Geometry check sheet. Reference: the model listing, model coordinates, mm. A direction names the side the tool comes from. Give positions to 0.01 mm unless a question says otherwise; leave off trailing zeros. Order: outer loops, then holes, each group sorted by start corner. A loop starts at its lowest first (then second) coordinate and runs counter-clockwise, first axis right, second up. Notation, with made-up numbers: M -30.75,76 L -11.75,76 A16 cw -11.75,91 Z; hole C -6.75,7 d11. An arc over 180 degrees is marked long. Answer as CSV lines item,"result".
from build123d import *

# Parameters (mm, degrees)
BOSS_EXTRUDE1_DEPTH = 21
BOSS_EXTRUDE2_DEPTH = 14
SKETCH6_R           = 2
CUT_EXTRUDE6_DEPTH  = 5
SKETCH7_R           = 2
CUT_EXTRUDE7_DEPTH  = 5


with BuildPart() as part:
    # Sketch2 → Boss-Extrude1 (new body)
    with BuildSketch(Plane.XY):
        with BuildLine():
            Line((-24, 0), (-14, 0))
            ThreePointArc((-14, 0), (-12.585786438, 0.585786438), (-12, 2))
            Line((-12, 2), (-12, 14))
            ThreePointArc((-12, 14), (-11.414213562, 15.414213562), (-10, 16))
            Line((-10, 16), (0, 16))
            Line((0, 16), (10, 16))
            ThreePointArc((10, 16), (11.414213562, 15.414213562), (12, 14))
            Line((12, 14), (12, 2))
            ThreePointArc((12, 2), (12.585786438, 0.585786438), (14, 0))
            Line((14, 0), (24, 0))
            Line((24, 0), (24, 2))
            Line((24, 2), (15, 2))
            ThreePointArc((15, 2), (14.292893219, 2.292893219), (14, 3))
            Line((14, 3), (14, 14))
            ThreePointArc((14, 14), (12.828427125, 16.828427125), (10, 18))
            Line((10, 18), (0, 18))
            Line((0, 18), (-10, 18))
            ThreePointArc((-10, 18), (-12.828427125, 16.828427125), (-14, 14))
            Line((-14, 14), (-14, 3))
            ThreePointArc((-14, 3), (-14.292893219, 2.292893219), (-15, 2))
            Line((-15, 2), (-24, 2))
            Line((-24, 2), (-24, 0))
        make_face()
    extrude(amount=BOSS_EXTRUDE1_DEPTH)

    # Sketch3 → Boss-Extrude2 (add)
    with BuildSketch(Plane.XY.offset(21)):
        with BuildLine():
            Line((-14, 3), (-12, 2))
            ThreePointArc((-12, 2), (-12.585786438, 0.585786438), (-14, 0))
            Line((-14, 0), (-24, 0))
            Line((-24, 0), (-24, 2))
            Line((-24, 2), (-15, 2))
            ThreePointArc((-15, 2), (-14.292893219, 2.292893219), (-14, 3))
        make_face()
        with BuildLine():
            Line((12, 2), (14, 3))
            ThreePointArc((14, 3), (14.292893219, 2.292893219), (15, 2))
            Line((15, 2), (24, 2))
            Line((24, 2), (24, 0))
            Line((24, 0), (14, 0))
            ThreePointArc((14, 0), (12.585786438, 0.585786438), (12, 2))
        make_face()
    extrude(amount=BOSS_EXTRUDE2_DEPTH)

    # Sketch6 → Cut-Extrude6 (cut)
    with BuildSketch(Plane(origin=(0, 0, 0), x_dir=(1, 0, 0), z_dir=(0, 1, 0))):
        with Locations(Location((-19, -5, 0), (0, 0, 90))):
            Circle(SKETCH6_R)
        with Locations(Location((-19, -30, 0), (0, 0, 90))):
            Circle(SKETCH6_R)
        with Locations(Location((19, -30, 0), (0, 0, 90))):
            Circle(SKETCH6_R)
        with Locations(Location((19, -5, 0), (0, 0, 90))):
            Circle(SKETCH6_R)
    extrude(amount=CUT_EXTRUDE6_DEPTH, mode=Mode.SUBTRACT)

    # Sketch7 → Cut-Extrude7 (cut)
    with BuildSketch(Plane(origin=(0, 18, 0), x_dir=(1, 0, 0), z_dir=(0, 1, 0))):
        with Locations(Location((0, -8, 0), (0, 0, 270))):
            Circle(SKETCH7_R)
        with Locations(Location((0, -16, 0), (0, 0, 270))):
            Circle(SKETCH7_R)
    extrude(amount=-CUT_EXTRUDE7_DEPTH, mode=Mode.SUBTRACT)


solid = part.part
(1) Section check B-B on x = 0. Enter the section's corners in (y, z), then the cut area to 3 significant figures.
The answers:
outline,"M 16,0 L 18,0 L 18,6 L 16,6 Z; M 16,10 L 18,10 L 18,14 L 16,14 Z; M 16,18 L 18,18 L 18,21 L 16,21 Z"
area,"26.0 mm2"
(2) Gauge pin test, flat ends, axial feed: P1, Ø7, axis at x = 21.5, z = 15, coming from the +Y side; P2, Ø3.5, axis at y = 9, z = 11, coming from the +X side; P3, Ø6, axis at x = -1.5, z = 8, coming from the -Y side; P4, Ø2.5, axis at x = 19, z = 5, coming from the +Y side. Record the tip position at first contact, or that the pin passes through.
The answers:
P1,"stops at y = 2"
P2,"stops at x = 14"
P3,"stops at y = 16"
P4,"passes through"
(3) Section check D-D on y = 6.75. Enter the section's corners in (x, z), then the cut area to 3 significant figures.
The answers:
outline,"M -14,0 L -12,0 L -12,21 L -14,21 Z; M 12,0 L 14,0 L 14,21 L 12,21 Z"
area,"84.0 mm2"
(4) Section check A-A on z = 16. Enter the section's corners in (x, y).
The answers:
outline,"M -24,0 L -14,0 A2 ccw -12,2 L -12,14 A2 cw -10,16 L -2,16 L -2,18 L -10,18 A4 ccw -14,14 L -14,3 A1 cw -15,2 L -24,2 Z; M 2,16 L 10,16 A2 cw 12,14 L 12,2 A2 ccw 14,0 L 24,0 L 24,2 L 15,2 A1 cw 14,3 L 14,14 A4 ccw 10,18 L 2,18 Z"
(5) Draft check along Z on faces 1 (the face through (11.4, 15.43, 10.35)), 2 (the face through (-18, 1, 35)), 3 (the face through (0, 17, 6)), 4 (the face through (-21, 1, 5)). Enter one of: +Z half, -Z half, draft (parallel to the pull), parting line (faces both ways), or undercut.
The answers:
face 1,"draft"
face 2,"+Z half"
face 3,"undercut"
face 4,"undercut"
(6) Section check C-C on z = 5. Enter the section's corners in (x, y), then the cut area to 3 significant figures.
The answers:
outline,"M -24,0 L -21,0 L -21,2 L -24,2 Z; M -17,0 L -14,0 A2 ccw -12,2 L -12,14 A2 cw -10,16 L 10,16 A2 cw 12,14 L 12,2 A2 ccw 14,0 L 17,0 L 17,2 L 15,2 A1 cw 14,3 L 14,14 A4 ccw 10,18 L -10,18 A4 ccw -14,14 L -14,3 A1 cw -15,2 L -17,2 Z; M 21,0 L 24,0 L 24,2 L 21,2 Z"
area,"138 mm2"
(7) Material ranges on line 1 (Z direction, x = -19, y = 0.6); line 2 (X direction, y = 13.5, z = 16.5); line 3 (Z direction, x = 18, y = 1.25), recorded low to high.
The answers:
line 1,"z = 0 to 3, 7 to 28, 32 to 35"
line 2,"x = -14 to -12, 12 to 14"
line 3,"z = 0 to 3.27, 6.73 to 28.27, 31.73 to 35"
(8) Tool access check on faces 5 (the face through (13, 2.5, 27.9)), 6 (the face through (14, 8, 10)), 7 (the face through (-12.57, 0.6, 17.26)). Record the directions out of +Z, -Z, +X, -X, +Y, -Y that give a thin tool (end or side, any length) a straight path to the whole face; none if there is none.
The answers:
face 5,"+Z, +Y"
face 6,"+Z, -Z, +X, +Y"
face 7,"+Z, -Z, -Y"
